```python
from build123d import *

# Parameters (mm, degrees)
SKETCH1_W           = 100
SKETCH1_H           = 30
BOSS_EXTRUDE1_DEPTH = 12.7
SKETCH2_W           = 15.2
SKETCH2_H           = 7.62
CUT_EXTRUDE1_DEPTH  = 102.913149299
SKETCH3_W           = 0.635
SKETCH3_H           = 5.08
SKETCH3_W_2         = 10.12
SKETCH3_H_2         = 0.635
CUT_EXTRUDE2_DEPTH  = 102.913149299
BOSS_EXTRUDE2_REACH = 103.913
SKETCH4_W           = 5
SKETCH4_H           = 16.47
FILLET7_R           = 1.5875
FILLET8_R           = 1.5875
BOSS_EXTRUDE3_REACH = 103.405
SKETCH9_W           = 19.05
SKETCH9_H           = 10.12
SKETCH7_R           = 2.54
CUT_EXTRUDE4_DEPTH  = 102.405445613
SKETCH10_R          = 3.429
CUT_EXTRUDE6_DEPTH  = 1.27
FILLET5_R           = 1.5875
BOSS_EXTRUDE4_DEPTH = 12.7
SKETCH12_R          = 4.5
CUT_EXTRUDE7_DEPTH  = 5.08
SKETCH13_R          = 2.75
CUT_EXTRUDE8_DEPTH  = 104.218974152
FILLET6_R           = 5
CUT_EXTRUDE9_START  = -1.27
CUT_EXTRUDE9_DEPTH  = 1.27
SKETCH25_W          = 3.175
SKETCH25_H          = 2.54
BOSS_EXTRUDE5_DEPTH = 2.54
BOSS_EXTRUDE6_REACH = 82.186
SKETCH26_W          = 2.54
SKETCH26_H          = 2.54
SKETCH31_W          = 0.1651
SKETCH31_H          = 2.54
ADJUST_DEPTH        = 72.14
FILLET9_R           = 1.5875


with BuildPart() as part:
    # Sketch1 → Boss-Extrude1 (new body)
    with BuildSketch(Plane(origin=(0, 0, 0), x_dir=(1, 0, 0), z_dir=(0, 1, 0))):
        with Locations((50, 0)):
            Rectangle(SKETCH1_W, SKETCH1_H)
    extrude(amount=BOSS_EXTRUDE1_DEPTH)

    # Sketch2 → Cut-Extrude1 (cut, through all)
    with BuildSketch(Plane(origin=(100, 0, 0), x_dir=(0, 0, -1), z_dir=(1, 0, 0))):
        with Locations((0, 3.81)):
            Rectangle(SKETCH2_W, SKETCH2_H)
    extrude(amount=-CUT_EXTRUDE1_DEPTH, mode=Mode.SUBTRACT)

    # Sketch3 → Cut-Extrude2 (cut, through all)
    with BuildSketch(Plane(origin=(100, 0, 0), x_dir=(0, 0, -1), z_dir=(1, 0, 0))):
        with Locations((-7.9175, 2.54)):
            Rectangle(SKETCH3_W, SKETCH3_H)
        with Locations((0, 7.9375)):
            Rectangle(SKETCH3_W_2, SKETCH3_H_2)
        with Locations((7.9175, 2.54)):
            Rectangle(SKETCH3_W, SKETCH3_H)
    extrude(amount=-CUT_EXTRUDE2_DEPTH, mode=Mode.SUBTRACT)

    # Sketch4 → Boss-Extrude2 (add, up to next)
    with BuildSketch(Plane.XZ, mode=Mode.PRIVATE) as boss_extrude2_sk1:
        with Locations((2.5, 0)):
            Rectangle(SKETCH4_W, SKETCH4_H)
    boss_extrude2_tool1 = extrude(boss_extrude2_sk1.sketch, amount=-BOSS_EXTRUDE2_REACH, mode=Mode.PRIVATE) - part.part
    add(boss_extrude2_tool1.solids().sort_by_distance((2.5, 0, 0))[0])

    # Fillet7
    fillet7_edges = [part.edges().sort_by_distance(p)[0] for p in [
        (5, 6.35, 7.6),
        (5, 6.35, -7.6),
    ]]
    fillet(fillet7_edges, radius=FILLET7_R)

    # Fillet8
    fillet8_edges = [part.edges().sort_by_distance(p)[0] for p in [
        (5, 2.54, 8.235),
        (5, 2.54, -8.235),
    ]]
    fillet(fillet8_edges, radius=FILLET8_R)

    # Sketch9 → Boss-Extrude3 (add, up to next)
    with BuildSketch(Plane.XZ.offset(-7.62), mode=Mode.PRIVATE) as boss_extrude3_sk1:
        with Locations((14.525, 0)):
            Rectangle(SKETCH9_W, SKETCH9_H)
    boss_extrude3_tool1 = extrude(boss_extrude3_sk1.sketch, amount=-BOSS_EXTRUDE3_REACH, mode=Mode.PRIVATE) - part.part
    add(boss_extrude3_tool1.solids().sort_by_distance((14.525, 7.62, 0))[0])

    # Sketch7 → Cut-Extrude4 (cut, through all)
    with BuildSketch(Plane.XZ.offset(-7.62)):
        with Locations(Location((13, 0, 0), (0, 0, 270))):
            Circle(SKETCH7_R)
    extrude(amount=-CUT_EXTRUDE4_DEPTH, mode=Mode.SUBTRACT)

    # Sketch10 → Cut-Extrude6 (cut)
    with BuildSketch(Plane.XZ.offset(-7.62)):
        with Locations(Location((13, 0, 0), (0, 0, 270))):
            Circle(SKETCH10_R)
    extrude(amount=-CUT_EXTRUDE6_DEPTH, mode=Mode.SUBTRACT)

    # Fillet5
    fillet5_edges = [part.edges().sort_by_distance(p)[0] for p in [
        (24.05, 7.9375, 5.06),
        (24.05, 7.9375, -5.06),
    ]]
    fillet(fillet5_edges, radius=FILLET5_R)

    # Sketch11 → Boss-Extrude4 (add)
    with BuildSketch(Plane(origin=(0, 12.7, 0), x_dir=(1, 0, 0), z_dir=(0, 1, 0))):
        with BuildLine():
            Line((73, -15), (73.022061133, -18.415))
            ThreePointArc((73.022061133, -18.415), (79.022061133, -24.415), (85.022061133, -18.415))
            Line((85.022061133, -18.415), (85, -15))
            Line((85, -15), (73, -15))
        make_face()
        with BuildLine():
            Line((27, -15.5), (27, -15))
            Line((27, -15), (15, -15))
            Line((15, -15), (15, -15.5))
            ThreePointArc((15, -15.5), (21, -21.5), (27, -15.5))
        make_face()
    boss_extrude4 = extrude(amount=-BOSS_EXTRUDE4_DEPTH)

    # Sketch12 → Cut-Extrude7 (cut)
    with BuildSketch(Plane(origin=(0, 12.7, 0), x_dir=(1, 0, 0), z_dir=(0, 1, 0))):
        with Locations(Location((21, -15.5, 0), (0, 0, 270))):
            Circle(SKETCH12_R)
        with Locations(Location((79.022061133, -18.415, 0), (0, 0, 270))):
            Circle(SKETCH12_R)
    cut_extrude7 = extrude(amount=-CUT_EXTRUDE7_DEPTH, mode=Mode.SUBTRACT)

    # Sketch13 → Cut-Extrude8 (cut, through all)
    with BuildSketch(Plane(origin=(0, 7.62, 0), x_dir=(1, 0, 0), z_dir=(0, 1, 0))):
        with Locations(Location((21, -15.5, 0), (0, 0, 270))):
            Circle(SKETCH13_R)
        with Locations(Location((79.022061133, -18.415, 0), (0, 0, 270))):
            Circle(SKETCH13_R)
    cut_extrude8 = extrude(amount=-CUT_EXTRUDE8_DEPTH, mode=Mode.SUBTRACT)

    # Mirror1: Boss-Extrude4, Cut-Extrude7, Cut-Extrude8 across plane
    add(boss_extrude4.mirror(Plane.XY))
    add(cut_extrude7.mirror(Plane.XY), mode=Mode.SUBTRACT)
    add(cut_extrude8.mirror(Plane.XY), mode=Mode.SUBTRACT)

    # Fillet6
    fillet6_edges = [part.edges().sort_by_distance(p)[0] for p in [
        (15, 6.35, 15),
        (27, 6.35, 15),
        (73, 6.35, 15),
        (85, 6.35, 15),
        (85, 6.35, -15),
        (73, 6.35, -15),
        (15, 6.35, -15),
        (27, 6.35, -15),
    ]]
    fillet(fillet6_edges, radius=FILLET6_R)

    # Sketch24 → Cut-Extrude9 (cut)
    with BuildSketch(Plane.XZ.offset(CUT_EXTRUDE9_START)):
        with BuildLine():
            Line((100, -10.775), (6.5875, -10.775))
            ThreePointArc((6.5875, -10.775), (3.668916761, -9.566083239), (2.46, -6.6475))
            Line((2.46, -6.6475), (2.46, 6.6475))
            ThreePointArc((2.46, 6.6475), (3.668916761, 9.566083239), (6.5875, 10.775))
            Line((6.5875, 10.775), (100, 10.775))
            Line((100, 10.775), (100, 15))
            Line((100, 15), (89.907270135, 15))
            ThreePointArc((89.907270135, 15), (86.636358391, 16.218315671), (84.959447861, 19.279545455))
            ThreePointArc((84.959447861, 19.279545455), (79.022061133, 24.415), (73.084674406, 19.279545455))
            ThreePointArc((73.084674406, 19.279545455), (71.407763876, 16.218315671), (68.136852132, 15))
            Line((68.136852132, 15), (31.03742995, 15))
            ThreePointArc((31.03742995, 15), (28.319643417, 15.803139702), (26.474961791, 17.954545455))
            ThreePointArc((26.474961791, 17.954545455), (21, 21.5), (15.525038209, 17.954545455))
            ThreePointArc((15.525038209, 17.954545455), (13.680356583, 15.803139702), (10.96257005, 15))
            Line((10.96257005, 15), (0, 15))
            Line((0, 15), (0, -15))
            Line((0, -15), (10.96257005, -15))
            ThreePointArc((10.96257005, -15), (13.680356583, -15.803139702), (15.525038209, -17.954545455))
            ThreePointArc((15.525038209, -17.954545455), (21, -21.5), (26.474961791, -17.954545455))
            ThreePointArc((26.474961791, -17.954545455), (28.319643417, -15.803139702), (31.03742995, -15))
            Line((31.03742995, -15), (68.136852132, -15))
            ThreePointArc((68.136852132, -15), (71.407763876, -16.218315671), (73.084674406, -19.279545455))
            ThreePointArc((73.084674406, -19.279545455), (79.022061133, -24.415), (84.959447861, -19.279545455))
            ThreePointArc((84.959447861, -19.279545455), (86.636358391, -16.218315671), (89.907270135, -15))
            Line((89.907270135, -15), (100, -15))
            Line((100, -15), (100, -10.775))
        make_face()
    extrude(amount=CUT_EXTRUDE9_DEPTH, mode=Mode.SUBTRACT)

    # Sketch25 → Boss-Extrude5 (add)
    with BuildSketch(Plane.XZ.offset(-7.62)):
        with Locations((26.2725, 6.33)):
            Rectangle(SKETCH25_W, SKETCH25_H)
        with Locations((26.2725, -6.33)):
            Rectangle(SKETCH25_W, SKETCH25_H)
    extrude(amount=BOSS_EXTRUDE5_DEPTH)

    # Sketch26 → Boss-Extrude6 (add, up to next)
    with BuildSketch(Plane.ZY.offset(-24.685), mode=Mode.PRIVATE) as boss_extrude6_sk1:
        with Locations((6.33, 6.35)):
            Rectangle(SKETCH26_W, SKETCH26_H)
    boss_extrude6_tool1 = extrude(boss_extrude6_sk1.sketch, amount=BOSS_EXTRUDE6_REACH, mode=Mode.PRIVATE) - part.part
    # Sketch26 → Boss-Extrude6 (add, up to next)
    with BuildSketch(Plane.ZY.offset(-24.685), mode=Mode.PRIVATE) as boss_extrude6_sk2:
        with Locations((-6.33, 6.35)):
            Rectangle(SKETCH26_W, SKETCH26_H)
    boss_extrude6_tool2 = extrude(boss_extrude6_sk2.sketch, amount=BOSS_EXTRUDE6_REACH, mode=Mode.PRIVATE) - part.part
    add(boss_extrude6_tool1.solids().sort_by_distance((24.685, 6.35, 6.33))[0])
    add(boss_extrude6_tool2.solids().sort_by_distance((24.685, 6.35, -6.33))[0])

    # Sketch31 → adjust (cut)
    with BuildSketch(Plane(origin=(100, 0, 0), x_dir=(0, 0, -1), z_dir=(1, 0, 0))):
        with Locations((7.68255, 6.35)):
            Rectangle(SKETCH31_W, SKETCH31_H)
        with Locations((-7.68255, 6.35)):
            Rectangle(SKETCH31_W, SKETCH31_H)
    extrude(amount=-ADJUST_DEPTH, mode=Mode.SUBTRACT)

    # Fillet9
    fillet9_edges = [part.edges().sort_by_distance(p)[0] for p in [
        (5, 6.35, 5.06),
        (5, 6.35, -5.06),
        (27.86, 6.35, 7.7651),
        (27.86, 6.35, -7.7651),
    ]]
    fillet(fillet9_edges, radius=FILLET9_R)


solid = part.part
```
Can you work these out from the model? Positions are in its coordinate system, mm. A direction names the side the tool comes from. Give positions to 0.01 mm unless a question says otherwise; leave off trailing zeros. Loops run counter-clockwise (first coordinate to the right, second up) from the corner with the lowest first, then second, coordinate; pieces in that order, holes last. Notation, with made-up numbers: M 85,35.5 L 126,35.5 A27 ccw 126,69.5 Z; hole C -11,-36.75 d6. An arc over 180 degrees is marked long. One line per item, written item: value.
(1) Suppose I cut it at C-C on x = 51. List the corners of the cut face in (y, z) for me (3 decimals).
Returned:
outline: M 0,-10.775 L 1.27,-10.775 L 1.27,-15 L 12.7,-15 L 12.7,15 L 1.27,15 L 1.27,10.775 L 0,10.775 L 0,8.235 L 5.08,8.235 L 5.08,7.765 L 7.62,7.765 L 7.62,5.06 L 8.255,5.06 L 8.255,-5.06 L 7.62,-5.06 L 7.62,-7.765 L 5.08,-7.765 L 5.08,-8.235 L 0,-8.235 Z
(2) I need wall thicknesses on line 1 (X direction, y = 12, z = -14.5); line 2 (Z direction, x = 35, y = 3.75) (3 decimals); line 3 (Z direction, x = 90.5, y = 6). Which ranges of each line are inside material? Lowest first, please.
Returned:
line 1: 0 to 16.61, 25.39 to 76.8, 81.24 to 100
line 2: -15 to -8.235, 8.235 to 15
line 3: -15 to -7.77, 7.77 to 15
(3) Suppose I cut it at B-B on z = 0. List the corners of the cut face in (x, y) for me (3 decimals).
Returned:
outline: M 0,1.27 L 2.46,1.27 L 2.46,0 L 5,0 L 5,7.62 L 9.571,7.62 L 9.571,8.89 L 10.46,8.89 L 10.46,12.7 L 0,12.7 Z; M 15.54,8.89 L 16.429,8.89 L 16.429,7.62 L 24.05,7.62 L 24.05,8.255 L 100,8.255 L 100,12.7 L 15.54,12.7 Z
(4) Will these pins go through, and if not, where does the flat tip stop? pin 1 (1 mm diameter, centred on y = 0.5, z = -2.5, fed in from -X); pin 2 (4 mm diameter, centred on x = 35, y = 8, fed in from -Z); pin 3 (4 mm diameter, centred on x = 19.5, z = 15.5, fed in from -Y); pin 4 (3 mm diameter, centred on x = 62, z = 7, fed in from -Y).
Returned:
pin 1: x = 2.46
pin 2: z = -15
pin 3: y = 1.27
pin 4: y = 0
(5) We'd pull the mould along Z, two halves only. Please class faces 4 (the face through (78.902, 7.065, 24.414)), 5 (the face through (54, 3, 8.235)), 6 (the face through (3.701, 0.644, -9.598)), 7 (the face through (100, 9, 0)): released by +Z, released by -Z, zero draft, split by the parting line, or undercut.
Returned:
face 4: released by +Z
face 5: undercut
face 6: released by -Z
face 7: zero draft
(6) Which directions (+Z, -Z, +X, -X, +Y, -Y) give clear straight access to the entire face, cutting with the end or side of a thin tool? Please do faces 1 (the face through (32, 5.08, -8)), 2 (the face through (49, 7, 15)), 3 (the face through (79.22, 10.2, -13.92)).
Returned:
face 1: +X, -Y
face 2: +Z, +Y, -Y
face 3: +Y
(7) Suppose I cut it at A-A on x = 21. Count the separate pieces of the cut face and the enclosed holes in it, plus the area to 3 significant figures.
Returned:
separate pieces: 3
enclosed holes: 0
area: 248 mm^2
